The model under review builds one solid part; all positions refer to its coordinate system, in mm. A direction names the side the tool comes from. Give positions to 0.01 mm unless a question says otherwise; leave off trailing zeros. Loops run counter-clockwise (first coordinate to the right, second up) from the corner with the lowest first, then second, coordinate; pieces in that order, holes last. Notation, with made-up numbers: (74, -12) - (126, -12) arc R17 ccw to (126, -5) - close; hole circle Ø7 at (-32, -14.5). An arc over 180 degrees is marked (long way). Return JSON: item names as keys, results as strings. Group by question number.
from build123d import *

# Parameters (mm, degrees)
SKETCH1_R           = 9.625
BOSS_EXTRUDE1_DEPTH = 0.625
SKETCH2_R           = 1.225
BOSS_EXTRUDE2_DEPTH = 85
BOSS_EXTRUDE3_DEPTH = 2.4
SKETCH4_R           = 1.25
CUT_EXTRUDE1_DEPTH  = 10


with BuildPart() as part:
    # Sketch1 → Boss-Extrude1 (new, symmetric)
    with BuildSketch(Plane.XY):
        Circle(SKETCH1_R)
    extrude(amount=BOSS_EXTRUDE1_DEPTH, both=True)

    # Sketch2 → Boss-Extrude2 (add)
    with BuildSketch(Plane.XY.offset(0.625)):
        Circle(SKETCH2_R)
    extrude(amount=BOSS_EXTRUDE2_DEPTH)

    # Sketch3 → Boss-Extrude3 (add, symmetric)
    with BuildSketch(Plane(origin=(0, 0, 0), x_dir=(0, 0, -1), z_dir=(1, 0, 0))):
        with BuildLine():
            Line((-85.625, 5), (-85.625, -5))
            Line((-85.625, -5), (-95.625, -5))
            ThreePointArc((-95.625, -5), (-100.625, 0), (-95.625, 5))
            Line((-95.625, 5), (-85.625, 5))
        make_face()
    extrude(amount=BOSS_EXTRUDE3_DEPTH, both=True)

    # Sketch4 → Cut-Extrude1 (cut)
    with BuildSketch(Plane.ZY.offset(2.4)):
        with Locations((95.625, 0)):
            Circle(SKETCH4_R)
    extrude(amount=-CUT_EXTRUDE1_DEPTH, mode=Mode.SUBTRACT)


solid = part.part
Item 1: Tool access review of faces 5 (the face through (2.4, 0, 93)), 6 (the face through (-7.638, -5.857, 0.009)), 7 (the face through (-2.4, 0, 93)), 8 (the face through (1, 1, 85.625)), 9 (the face through (0, -5, 91)): name each direction out of +Z, -Z, +X, -X, +Y, -Y from which nothing blocks a thin tool from reaching the whole face with its end or side.
Item 2: Take a section at C-C (z = 87). State the section outline as (x, y) points.
Item 3: Take a section at D-D (x = -7.75). State the section outline as (y, z) points (3 decimals), then the cut area to 3 significant figures.
Item 4: Take a section at B-B (x = 0). State the section outline as (y, z) points (3 decimals).
Item 5: For L1, parallel to Z at x = 4, y = 4.75 (3 decimals); L2, parallel to Z at x = 2, y = -2.5 (3 decimals); L3, parallel to Z at x = 0.75, y = 1.75 (3 decimals), list the stretches that pass through material, from the lowest coordinate up. Write a range as from..to.
Item 6: Take a section at A-A (y = 0). State the section outline as (x, z) points (3 decimals).
Item 7: For P1, Ø5.5, axis at x = 1, z = 89.5, coming from the +Y side; P2, Ø4, axis at x = -1.5, z = 66.5, coming from the +Y side (3 decimals); P3, Ø11, axis at y = 1, z = 90, coming from the -X side, all flat-tipped, find the tip position at first contact; note any pin that passes through.
Item 8: Mouldability with a two-part tool opening along Z and no side actions: class faces 1 (the face through (0, 0, -0.625)), 2 (the face through (0, 5, 91)), 3 (the face through (-0.034, 0.375, 96.817)), 4 (the face through (-0.266, -1.196, 42.53)) as +Z half, -Z half, draft (parallel to the pull), parting line (faces both ways), or undercut.
Check sheet entries:
{
 "1": {"face 5": "+Z, +X, +Y, -Y", "face 6": "+Z, -Z", "face 7": "+Z, -X, +Y, -Y", "face 8": "none", "face 9": "+Z, +X, -X, -Y"},
 "2": {"outline": "(-2.4, -5) - (2.4, -5) - (2.4, 5) - (-2.4, 5) - close"},
 "3": {"outline": "(-5.708, -0.625) - (5.708, -0.625) - (5.708, 0.625) - (-5.708, 0.625) - close", "area": "14.3 mm^2"},
 "4": {"outline": "(-9.625, -0.625) - (9.625, -0.625) - (9.625, 0.625) - (1.225, 0.625) - (1.225, 85.625) - (5, 85.625) - (5, 95.625) arc R5 ccw to (-5, 95.625) - (-5, 85.625) - (-1.225, 85.625) - (-1.225, 0.625) - (-9.625, 0.625) - close; hole circle Ø2.5 at (0, 95.625)"},
 "5": {"L1": "z = -0.625..0.625", "L2": "z = -0.625..0.625, 85.625..99.955", "L3": "z = -0.625..0.625, 85.625..100.309"},
 "6": {"outline": "(-9.625, -0.625) - (9.625, -0.625) - (9.625, 0.625) - (1.225, 0.625) - (1.225, 85.625) - (2.4, 85.625) - (2.4, 94.375) - (-2.4, 94.375) - (-2.4, 85.625) - (-1.225, 85.625) - (-1.225, 0.625) - (-9.625, 0.625) - close; (-2.4, 96.875) - (2.4, 96.875) - (2.4, 100.625) - (-2.4, 100.625) - close"},
 "7": {"P1": "stops at y = 5", "P2": "stops at y = 1.225", "P3": "stops at x = -2.4"},
 "8": {"face 1": "-Z half", "face 2": "draft", "face 3": "undercut", "face 4": "undercut"}
}
